from build123d import *

# Parameters (mm, degrees)
SKETCH1_R           = 2
BOSS_EXTRUDE1_DEPTH = 10
CUT_EXTRUDE3_REACH  = 25.585
SKETCH2_W           = 8
SKETCH2_H           = 5.25
SKETCH3_W           = 17
SKETCH3_H           = 12
CUT_EXTRUDE4_DEPTH  = 10
FILLET1_R           = 2


with BuildPart() as part:
    # Sketch1 → Boss-Extrude1 (new, symmetric)
    with BuildSketch(Plane.XY):
        with BuildLine():
            Line((17.5, -3), (-17.5, -3))
            ThreePointArc((-17.5, -3), (-20.5, 0), (-17.5, 3))
            Line((-17.5, 3), (17.5, 3))
            ThreePointArc((17.5, 3), (20.5, 0), (17.5, -3))
        make_face()
        with Locations((17.5, 0)):
            Circle(SKETCH1_R, mode=Mode.SUBTRACT)
        with Locations((-17.5, 0)):
            Circle(SKETCH1_R, mode=Mode.SUBTRACT)
    extrude(amount=BOSS_EXTRUDE1_DEPTH, both=True)

    # Cut-Extrude3: up to this face of the body (flat: up to its plane)
    cut_extrude3_end = Plane(part.part.faces().sort_by_distance((0, -3, 0))[0])
    # Sketch2 → Cut-Extrude3 (cut, up to the picked face)
    with BuildSketch(Plane(origin=(0, 3, 0), x_dir=(1, 0, 0), z_dir=(0, 1, 0)), mode=Mode.PRIVATE) as cut_extrude3_sk1:
        with Locations((-16.5, -7.375)):
            Rectangle(SKETCH2_W, SKETCH2_H)
    cut_extrude3_tool1 = split(extrude(cut_extrude3_sk1.sketch, amount=-CUT_EXTRUDE3_REACH, mode=Mode.PRIVATE), bisect_by=cut_extrude3_end, keep=Keep.BOTH, mode=Mode.PRIVATE)
    # Sketch2 → Cut-Extrude3 (cut, up to the picked face)
    with BuildSketch(Plane(origin=(0, 3, 0), x_dir=(1, 0, 0), z_dir=(0, 1, 0)), mode=Mode.PRIVATE) as cut_extrude3_sk2:
        with Locations((-16.5, 7.375)):
            Rectangle(SKETCH2_W, SKETCH2_H)
    cut_extrude3_tool2 = split(extrude(cut_extrude3_sk2.sketch, amount=-CUT_EXTRUDE3_REACH, mode=Mode.PRIVATE), bisect_by=cut_extrude3_end, keep=Keep.BOTH, mode=Mode.PRIVATE)
    # Sketch2 → Cut-Extrude3 (cut, up to the picked face)
    with BuildSketch(Plane(origin=(0, 3, 0), x_dir=(1, 0, 0), z_dir=(0, 1, 0)), mode=Mode.PRIVATE) as cut_extrude3_sk3:
        with Locations((16.5, 7.375)):
            Rectangle(SKETCH2_W, SKETCH2_H)
    cut_extrude3_tool3 = split(extrude(cut_extrude3_sk3.sketch, amount=-CUT_EXTRUDE3_REACH, mode=Mode.PRIVATE), bisect_by=cut_extrude3_end, keep=Keep.BOTH, mode=Mode.PRIVATE)
    # Sketch2 → Cut-Extrude3 (cut, up to the picked face)
    with BuildSketch(Plane(origin=(0, 3, 0), x_dir=(1, 0, 0), z_dir=(0, 1, 0)), mode=Mode.PRIVATE) as cut_extrude3_sk4:
        with Locations((16.5, -7.375)):
            Rectangle(SKETCH2_W, SKETCH2_H)
    cut_extrude3_tool4 = split(extrude(cut_extrude3_sk4.sketch, amount=-CUT_EXTRUDE3_REACH, mode=Mode.PRIVATE), bisect_by=cut_extrude3_end, keep=Keep.BOTH, mode=Mode.PRIVATE)
    add(cut_extrude3_tool1.solids().sort_by(Axis((-16.5, 3, 7.375), (0, -1, 0)))[0], mode=Mode.SUBTRACT)
    add(cut_extrude3_tool2.solids().sort_by(Axis((-16.5, 3, -7.375), (0, -1, 0)))[0], mode=Mode.SUBTRACT)
    add(cut_extrude3_tool3.solids().sort_by(Axis((16.5, 3, -7.375), (0, -1, 0)))[0], mode=Mode.SUBTRACT)
    add(cut_extrude3_tool4.solids().sort_by(Axis((16.5, 3, 7.375), (0, -1, 0)))[0], mode=Mode.SUBTRACT)

    # Sketch3 → Cut-Extrude4 (cut)
    with BuildSketch(Plane(origin=(0, 3, 0), x_dir=(1, 0, 0), z_dir=(0, 1, 0))):
        Rectangle(SKETCH3_W, SKETCH3_H)
    extrude(amount=-CUT_EXTRUDE4_DEPTH, mode=Mode.SUBTRACT)

    # Fillet1
    fillet1_edges = [part.edges().sort_by_distance(p)[0] for p in [
        (-8.5, 0, 6),
        (-8.5, 0, -6),
        (8.5, 0, -6),
        (8.5, 0, 6),
    ]]
    fillet(fillet1_edges, radius=FILLET1_R)


solid = part.part
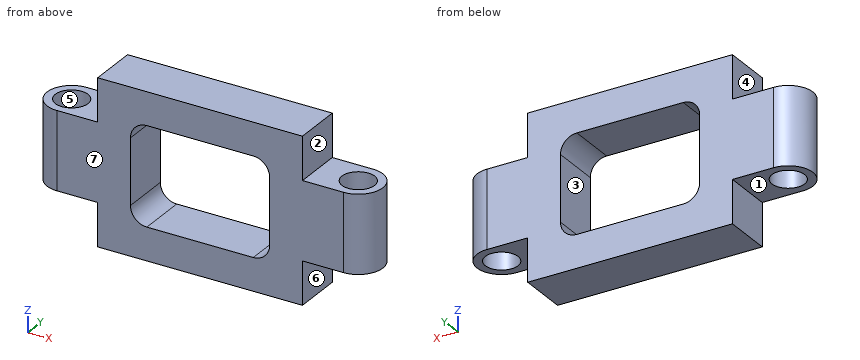
The listing builds one solid part. Answer for the finished solid, in the listing's coordinates (mm). Face numbers are marked on the shaded views. A direction names the side the tool comes from. Coordinates: 2 decimals unless noted, no trailing zeros. Order: outer loops, then holes, each group sorted by start corner. A loop starts at its lowest first (then second) coordinate and runs counter-clockwise, first axis right, second up. Notation, with made-up numbers: (-9, 50.5) -> (13, 50.5) arc R28 ccw to (13, 72.5) -> close; hole circle Ø6 at (28.5, -12.5). An arc over 180 degrees is marked (long way). Answer in a Markdown table with one row per item. Add a question column.
Item 1: Each of these flat-tipped pins is pushed along its axis until it touches: P1, Ø2, axis at y = -1.5, z = -5, coming from the -X side; P2, Ø1.6, axis at y = 0, z = -8.5, coming from the -X side; P3, Ø3, axis at x = -14.5, y = -1, coming from the +Z side. Where does it stop, or does it pass through?
Item 2: Find section D-D (z = -5.5). Write down the section's boundary in (x, y), then the cut area to 3 significant figures.
Item 3: Determine the mould class of the marked faces 5, 6 and 7 for opening direction Y: +Y half, -Y half, draft (parallel to the pull), parting line (faces both ways), or undercut.
Item 4: Which of the six approach directions +Z, -Z, +X, -X, +Y, -Y give full straight-line access (tool end or side, diameter ignored) to the marked faces 1, 2, 3 and 4?
Item 5: Find section C-C (x = -5). Write down the section's boundary in (y, z), then the cut area to 3 significant figures.
Item 6: Find section B-B (z = -3.5). Write down the section's boundary in (x, y), then the cut area to 3 significant figures.
Item 7: Find section A-A (y = 0). Write down the section's boundary in (x, z), then the cut area to 3 significant figures.
Item 8: Find the intervals of material crossed by L1, parallel to X at y = 0, z = -1.5; L2, parallel to Y at x = 17.5, z = 2; L3, parallel to X at y = -1.2, z = 0.5, in increasing order. Write a range as from..to.
Result set:
| question | item | result |
|---|---|---|
| 1 | P1 | stops at x = -20.45 |
| 1 | P2 | stops at x = -12.5 |
| 1 | P3 | stops at z = 4.75 |
| 2 | outline | (-12.5, -3) -> (-7.82, -3) -> (-7.82, 3) -> (-12.5, 3) -> close; (7.82, -3) -> (12.5, -3) -> (12.5, 3) -> (7.82, 3) -> close |
| 2 | area | 56.1 mm² |
| 3 | face 5 | undercut |
| 3 | face 6 | draft |
| 3 | face 7 | -Y half |
| 4 | face 1 | -Z, -X, +Y, -Y |
| 4 | face 2 | +Z, +X, +Y, -Y |
| 4 | face 3 | +Y, -Y |
| 4 | face 4 | +Z, -X, +Y, -Y |
| 5 | outline | (-3, -10) -> (3, -10) -> (3, -6) -> (-3, -6) -> close; (-3, 6) -> (3, 6) -> (3, 10) -> (-3, 10) -> close |
| 5 | area | 48.0 mm² |
| 6 | outline | (-17.5, -3) -> (-8.5, -3) -> (-8.5, 3) -> (-17.5, 3) arc R3 ccw to start; (8.5, -3) -> (17.5, -3) arc R3 ccw to (17.5, 3) -> (8.5, 3) -> close; hole circle Ø4 at (-17.5, 0); hole circle Ø4 at (17.5, 0) |
| 6 | area | 111 mm² |
| 7 | outline | (-20.5, -4.75) -> (-19.5, -4.75) -> (-19.5, 4.75) -> (-20.5, 4.75) -> close; (-15.5, -4.75) -> (-12.5, -4.75) -> (-12.5, -10) -> (12.5, -10) -> (12.5, -4.75) -> (15.5, -4.75) -> (15.5, 4.75) -> (12.5, 4.75) -> (12.5, 10) -> (-12.5, 10) -> (-12.5, 4.75) -> (-15.5, 4.75) -> close; (19.5, -4.75) -> (20.5, -4.75) -> (20.5, 4.75) -> (19.5, 4.75) -> close; hole (-8.5, -4) arc R2 ccw to (-6.5, -6) -> (6.5, -6) arc R2 ccw to (8.5, -4) -> (8.5, 4) arc R2 ccw to (6.5, 6) -> (-6.5, 6) arc R2 ccw to (-8.5, 4) -> close |
| 7 | area | 375 mm² |
| 8 | L1 | x = -20.5..-19.5, -15.5..-8.5, 8.5..15.5, 19.5..20.5 |
| 8 | L2 | y = -3..-2, 2..3 |
| 8 | L3 | x = -20.25..-19.1, -15.9..-8.5, 8.5..15.9, 19.1..20.25 |
